Job drawing, mm, ordinate dimensions from the low corner. One solid piece. A direction names the side the tool comes from. Give positions to 0.01 mm unless a question says otherwise; leave off trailing zeros. Loops run counter-clockwise (first coordinate to the right, second up) from the corner with the lowest first, then second, coordinate; pieces in that order, holes last. Notation, with made-up numbers: (32.5, -39) - (58.5, -39) arc R30 ccw to (58.5, -17) - close; hole circle Ø6 at (81.25, -11.75). An arc over 180 degrees is marked (long way). Use a Markdown table: item, result.
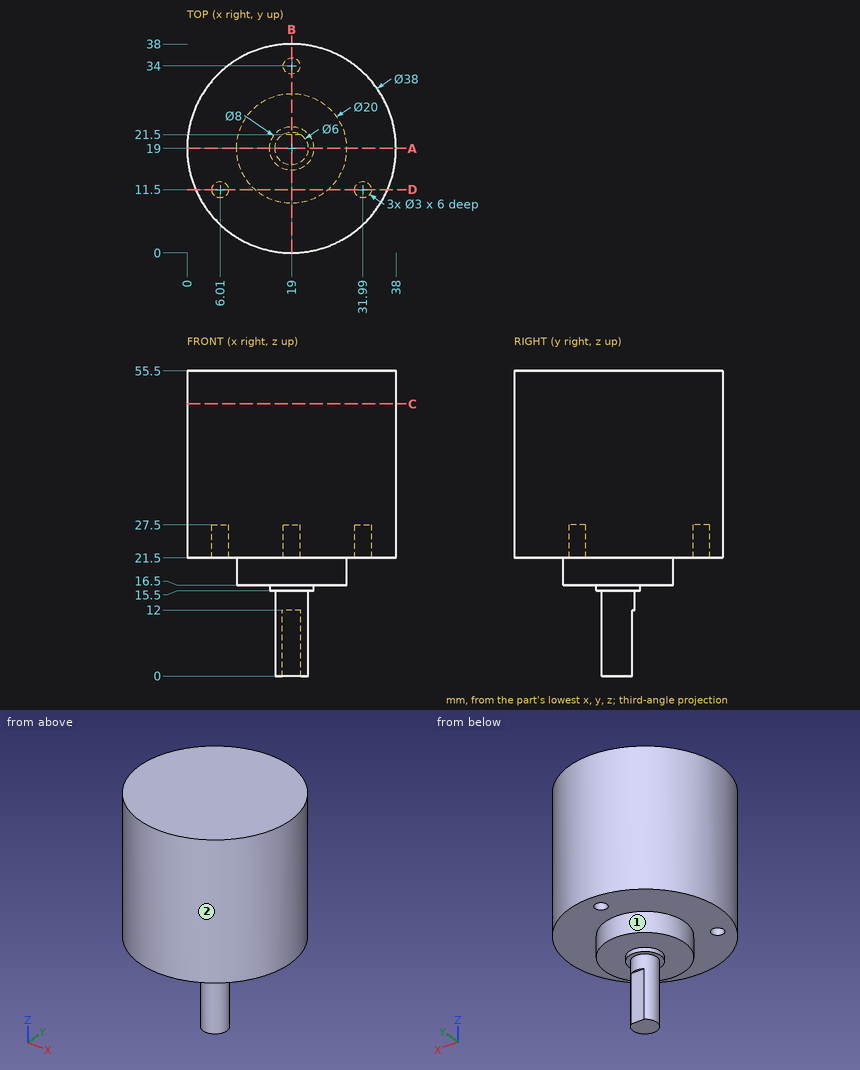
(1) Slice it at B-B, the plane x = 19. Write the cut outline in (y, z).
Computed:
| item | result |
|---|---|
| outline | (0, 21.5) - (9, 21.5) - (9, 16.5) - (15, 16.5) - (15, 15.5) - (16, 15.5) - (16, 0) - (21.5, 0) - (21.5, 12) - (22, 12) - (22, 15.5) - (23, 15.5) - (23, 16.5) - (29, 16.5) - (29, 21.5) - (32.5, 21.5) - (32.5, 27.5) - (35.5, 27.5) - (35.5, 21.5) - (38, 21.5) - (38, 55.5) - (0, 55.5) - close |
(2) Slice it at D-D, the plane y = 11.5. Write the cut outline in (x, z) (1 decimal), plus the area to 3 significant figures.
Computed:
| item | result |
|---|---|
| outline | (1.5, 21.5) - (4.5, 21.5) - (4.5, 27.5) - (7.5, 27.5) - (7.5, 21.5) - (12.4, 21.5) - (12.4, 16.5) - (25.6, 16.5) - (25.6, 21.5) - (30.5, 21.5) - (30.5, 27.5) - (33.5, 27.5) - (33.5, 21.5) - (36.5, 21.5) - (36.5, 55.5) - (1.5, 55.5) - close |
| area | 1,220 mm² |
(3) Slice it at C-C, the plane z = 49.5. Write the cut outline in (x, y).
Computed:
| item | result |
|---|---|
| outline | circle Ø38 at (19, 19) |
(4) 3-axis set-ups, long thin cutter, end or side, ignore diameter. For the marked faces 1 and 2: which of +Z, -Z, +X, -X, +Y, -Y reach the whole face in a straight line?
Computed:
| item | result |
|---|---|
| face 1 | -Z |
| face 2 | +Z, -Z |
(5) Drill centre lines: probe 1 along Y at (x, z) = (19, 25.85); probe 2 along X at (y, z) = (11, 23) (1 decimal); probe 3 along Z at (x, y) = (23, 18). Where is each one in solid material? Low to high. Write a range as [from, to].
Computed:
| item | result |
|---|---|
| probe 1 | [0, 32.5], [35.5, 38] |
| probe 2 | [1.8, 4.6], [7.4, 30.6], [33.4, 36.2] |
| probe 3 | [16.5, 55.5] |
(6) Slice it at A-A, the plane y = 19. Write the cut outline in (x, z).
Computed:
| item | result |
|---|---|
| outline | (0, 21.5) - (9, 21.5) - (9, 16.5) - (15, 16.5) - (15, 15.5) - (16, 15.5) - (16, 0) - (22, 0) - (22, 15.5) - (23, 15.5) - (23, 16.5) - (29, 16.5) - (29, 21.5) - (38, 21.5) - (38, 55.5) - (0, 55.5) - close |
(7) Pin check, flat tips, straight feed: P1, Ø3.5, axis at x = 19, y = 34, coming from the -Z side; P2, Ø8, axis at x = 25, z = 17, coming from the -Y side; P3, Ø4, axis at x = 19, z = 43, coming from the -Y side; P4, Ø10, axis at y = 30.5, z = 11.5, coming from the +X side (1 decimal). Stop position of each tip, or through.
Computed:
| item | result |
|---|---|
| P1 | z = 21.5 |
| P2 | y = 9.2 |
| P3 | y = 0 |
| P4 | through |
